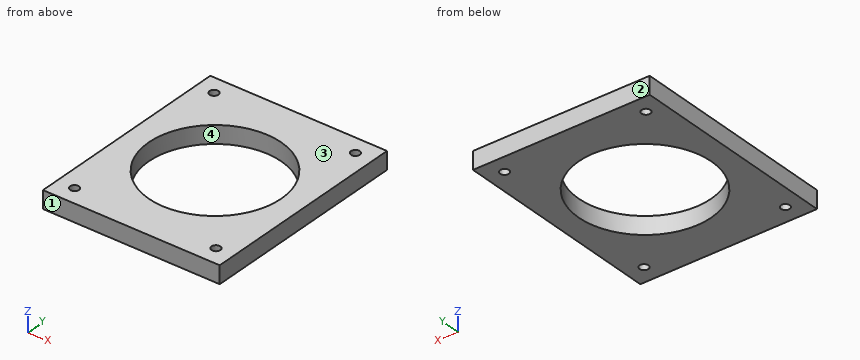
```python
from build123d import *

# Parameters (mm, degrees)
SKETCH1_W               = 127
SKETCH1_H               = 152.4
BOSS_EXTRUDE1_DEPTH     = 12.7
SKETCH2_R               = 47.625
CUT_EXTRUDE1_DEPTH      = 100.9999
CUT_EXTRUDE3_DEPTH      = 100.9999
CUT_EXTRUDE3_DEPTH_BACK = 100.9999
SKETCH3_R               = 3.175


with BuildPart() as part:
    # Sketch1 → Boss-Extrude1 (new body)
    with BuildSketch(Plane.XY):
        Rectangle(SKETCH1_W, SKETCH1_H)
    extrude(amount=BOSS_EXTRUDE1_DEPTH)

    # Sketch2 → Cut-Extrude1 (cut, through all)
    with BuildSketch(Plane(origin=(0, 0, 0), x_dir=(-1, 0, 0), z_dir=(0, 0, -1))):
        Circle(SKETCH2_R)
    extrude(amount=-CUT_EXTRUDE1_DEPTH, mode=Mode.SUBTRACT)

    # Sketch3 → Cut-Extrude3 (cut, two sides: drawn at the far end of the back side and taken through both)
    with BuildSketch(Plane(origin=(0, 0, 0), x_dir=(-1, 0, 0), z_dir=(0, 0, -1)).offset(-CUT_EXTRUDE3_DEPTH_BACK)):
        with Locations((-50.8, 63.5)):
            Circle(SKETCH3_R)
        with Locations((50.8, 63.5)):
            Circle(SKETCH3_R)
        with Locations((50.8, -63.5)):
            Circle(SKETCH3_R)
        with Locations((-50.8, -63.5)):
            Circle(SKETCH3_R)
    extrude(amount=CUT_EXTRUDE3_DEPTH + CUT_EXTRUDE3_DEPTH_BACK, mode=Mode.SUBTRACT)


solid = part.part
```
Verification items for the finished model (mm, model axes). Face numbers are marked on the shaded views. Give positions to 0.01 mm unless a question says otherwise; leave off trailing zeros. Order: outer loops, then holes, each group sorted by start corner. A loop starts at its lowest first (then second) coordinate and runs counter-clockwise, first axis right, second up. Notation, with made-up numbers: (-3, -39) - (17, -39) arc R12 ccw to (17, -20) - close; hole circle Ø6 at (28, -15). An arc over 180 degrees is marked (long way). Answer as CSV lines item,"result". Start each with the question number.
Item 1: Material ranges on L1, parallel to Y at x = -50.8, z = 5.25 (3 decimals); L2, parallel to X at y = -63.5, z = 7.25 (3 decimals); L3, parallel to Y at x = 53.5, z = 3, recorded low to high.
Item 2: Section check B-B, the plane z = 4. Record the boundary of the cut face in (x, y) (3 decimals).
Item 3: Section check C-C, the plane x = 50.8. Record the boundary of the cut face in (y, z) (3 decimals), plus the area to 3 significant figures.
Item 4: Section check D-D, the plane y = -63.5. Record the boundary of the cut face in (x, z) (3 decimals), plus the area to 3 significant figures.
Item 5: Section check A-A, the plane y = 0. Record the boundary of the cut face in (x, z) (3 decimals).
Item 6: Mould release check, pull along Y, two halves, no side actions. Record for the marked faces 1, 2, 3 and 4: released by +Y, released by -Y, zero draft, split by the parting line, or undercut.
Filled in:
1,L1,"-76.2 to -66.675, -60.325 to 60.325, 66.675 to 76.2"
1,L2,"-63.5 to -53.975, -47.625 to 47.625, 53.975 to 63.5"
1,L3,"-76.2 to -65.17, -61.83 to 61.83, 65.17 to 76.2"
2,outline,"(-63.5, -76.2) - (63.5, -76.2) - (63.5, 76.2) - (-63.5, 76.2) - close; hole circle Ø6.35 at (-50.8, -63.5); hole circle Ø6.35 at (-50.8, 63.5); hole circle Ø95.25 at (0, 0); hole circle Ø6.35 at (50.8, -63.5); hole circle Ø6.35 at (50.8, 63.5)"
3,outline,"(-76.2, 0) - (-66.675, 0) - (-66.675, 12.7) - (-76.2, 12.7) - close; (-60.325, 0) - (60.325, 0) - (60.325, 12.7) - (-60.325, 12.7) - close; (66.675, 0) - (76.2, 0) - (76.2, 12.7) - (66.675, 12.7) - close"
3,area,"1,770 mm^2"
4,outline,"(-63.5, 0) - (-53.975, 0) - (-53.975, 12.7) - (-63.5, 12.7) - close; (-47.625, 0) - (47.625, 0) - (47.625, 12.7) - (-47.625, 12.7) - close; (53.975, 0) - (63.5, 0) - (63.5, 12.7) - (53.975, 12.7) - close"
4,area,"1,450 mm^2"
5,outline,"(-63.5, 0) - (-47.625, 0) - (-47.625, 12.7) - (-63.5, 12.7) - close; (47.625, 0) - (63.5, 0) - (63.5, 12.7) - (47.625, 12.7) - close"
6,face 1,"released by -Y"
6,face 2,"released by +Y"
6,face 3,"zero draft"
6,face 4,"undercut"
